CAD build for the part. Positions are in the model's coordinates, mm. A direction names the side the tool comes from. Give positions to 0.01 mm unless a question says otherwise; leave off trailing zeros. Order: outer loops, then holes, each group sorted by start corner. A loop starts at its lowest first (then second) coordinate and runs counter-clockwise, first axis right, second up.
from build123d import *

# Parameters (mm, degrees)
F0_W     = 45
F0_H     = 25
F1_DEPTH = 250
F2_START = 250
F2_DEPTH = 50
F3_START = 280
F3_DEPTH = 20
F4_R     = 9.99999


# Not quite as in the source:
# - a fillet or chamfer is up to 0.001 mm smaller than in the source, because OpenCascade refuses the exact size


with BuildPart() as f1:
    # F0 (on Top) → F1 (new body)
    with BuildSketch(Plane.XY):
        Polygon((0, 380), (0, 0), (117.5, 0), (117.5, 25), (162.5, 25), (162.5, 0), (280, 0), (280, 380), align=None)
        with Locations((140, 12.5)):
            Rectangle(F0_W, F0_H)
    extrude(amount=F1_DEPTH)

    # F0 (on Top) → F2 (join)
    with BuildSketch(Plane.XY.offset(F2_START)):
        with Locations((140, 12.5)):
            Rectangle(F0_W, F0_H)
    extrude(amount=F2_DEPTH)

    # F0 (on Top) → F3 (join)
    with BuildSketch(Plane.XY.offset(F3_START)):
        Polygon((162.5, 0), (117.5, 0), (117.5, -116.4670363069), (140, -116.4670363069), (162.5, -116.4670363069), align=None)
    extrude(amount=F3_DEPTH)

    # F4 (radius 10 in the source; OpenCascade refuses exactly that, so slightly less here)
    f4_edges = [f1.edges().sort_by_distance(p)[0] for p in [
        (140, 25, 300),
        (117.5, -45.733518, 300),
        (162.5, -45.733518, 300),
        (162.5, 25, 275),
        (117.5, 25, 275),
        (162.5, -58.233518, 280),
        (117.5, -58.233518, 280),
        (162.5, 0, 265),
        (117.5, 0, 265),
        (117.5, -116.467036, 290),
        (140, -116.467036, 300),
        (162.5, -116.467036, 290),
        (140, -116.467036, 280),
    ]]
    fillet(f4_edges, radius=F4_R)


solid = f1.part
1. Saw through at C-C on z = 207. Give the cut face in (x, y).
2. Pin check, flat tips, straight feed: P1, Ø12, axis at x = 57.5, y = 324, coming from the +Z side; P2, Ø12.5, axis at x = 142.5, z = 275.5, coming from the +Y side; P3, Ø20, axis at x = 141, y = -76.5, coming from the -Z side. Stop position of each tip, or through.
3. Wall check: line 1 (Y direction, x = 262, z = 128.5); line 2 (Z direction, x = 129.5, y = 171.5); line 3 (X direction, y = 23.5, z = 265). Give the ranges that are in metal, low to high.
4. Saw through at B-B on x = 46. Give the cut face in (y, z).
5. Mould opens along Z. For faces 1 (the flat face through (138, 193, 0)), 2 (the flat face through (140, -45, 300)), 3 (the cylindrical face through (120.35, 3.01, 265.84)) say: released by +Z, released by -Z, zero draft, split by the parting line, or undercut.
6. 3-axis set-ups, long thin cutter, end or side, ignore diameter. For faces 4 (the cylindrical face through (120.35, 21.99, 270.28)), 5 (the cylindrical face through (159.65, 3.01, 265.84)), 6 (the cylindrical face through (159.65, 21.99, 270.28)), 7 (the flat face through (140, -52, 280)): which of +Z, -Z, +X, -X, +Y, -Y reach the whole face in a straight line?
Reported:
1. outline: (0, 0) - (280, 0) - (280, 380) - (0, 380) - close
2. P1: stops at z = 250
2. P2: stops at y = 25
2. P3: stops at z = 280
3. line 1: y = 0 to 380
3. line 2: z = 0 to 250
3. line 3: x = 122.23 to 157.77
4. outline: (0, 0) - (380, 0) - (380, 250) - (0, 250) - close
5. face 1: released by -Z
5. face 2: released by +Z
5. face 3: undercut
6. face 4: +Z, -X, +Y
6. face 5: +X, -Y
6. face 6: +Z, +X, +Y
6. face 7: -Z, +X, -X, -Y
